The listing builds one solid part. Answer for the finished solid, in the listing's coordinates (mm). Round coordinates to 2 decimals unless told otherwise and drop trailing zeros. Order: outer loops, then holes, each group sorted by start corner. A loop starts at its lowest first (then second) coordinate and runs counter-clockwise, first axis right, second up. Notation, with made-up numbers: (88, -25) -> (135, -25) arc R30 ccw to (135, 13) -> close; hole circle Ø1 at (10, 40). An arc over 180 degrees is marked (long way). Return JSON: item names as keys, results as strings. Group by question number.
(1) The part is cut by section C-C (y = -12). Determine the outline of the cut face in (x, z), plus the area to 3 significant figures.
(2) The part is cut by section A-A (y = 71). Determine the outline of the cut face in (x, z), plus the area to 3 significant figures.
(3) Determine the mould class of faces 1 (the face through (0, 68, 35)), 2 (the face through (3.13, -0.42, -20.64)), 3 (the face through (3.1, 43.4, 131.7)) for opening direction Y: +Y half, -Y half, draft (parallel to the pull), parting line (faces both ways), or undercut.
(4) Consider line 1 (Z direction, x = 1.75, y = 31.75); line 2 (Y direction, x = 2.5, z = -20); line 3 (Z direction, x = 4, y = -31.75). Determine where each line is inside the solid, lowest interval first. Write a range as [from, to].
(5) The part is cut by section B-B (z = 101.5). Determine the outline of the cut face in (x, y), plus the area to 3 significant figures.
(6) Each of these flat-tipped pins is pushed along its axis until it touches: pin 1 (1.5 mm diameter, centred on x = 2.5, y = 41, fed in from -Z); pin 2 (1 mm diameter, centred on x = 4.5, z = 69, fed in from +Y); pin 3 (4 mm diameter, centred on y = 31.75, z = -20.64, fed in from +X); pin 4 (3 mm diameter, centred on x = 2, z = 22, fed in from -Y). Where does it stop, or does it pass through?
Autodesk Inventor part; units mm, degrees
ref_plane "YZ Plane" through (0, 0, 0) normal (1, 0, 0) x (0, 1, 0)
ref_plane "XZ Plane" through (0, 0, 0) normal (0, 1, 0) x (-1, 0, 0)
ref_plane "XY Plane" through (0, 0, 0) normal (0, 0, 1) x (1, 0, 0)
sketch "Sketch1" plane through (0, 0, 0) normal (1, 0, 0) x (0, 1, 0)
  line L0 (31.75, 0) -> (-31.75, 0) construction
  line L1 (-31.75, 0) -> (-31.75, -20.6375) construction
  line L2 (31.75, -20.6375) -> (31.75, 20.6375) construction
  circle A0 centre (31.75, -20.6375) radius 3.175
  circle A1 centre (31.75, 20.6375) radius 3.175
  circle A2 centre (-31.75, -20.6375) radius 3.175
  arc A3 (32.3103, 26.9627) -> (31.75, 121.7883) centre (36.5125, 74.402) ccw
  arc A4 (32.3103, 26.9627) -> (26.7051, 24.4939) centre (31.75, 20.6375) ccw
  arc A5 (-33.2262, -14.4615) -> (-29.3077, -26.499) centre (-31.75, -20.6375) ccw
  arc A6 (-33.2262, -14.4615) -> (26.7051, 24.4939) centre (-58.0173, 89.2573) ccw
  arc A7 (29.3077, -26.499) -> (37.057, -24.1244) centre (31.75, -20.6375) ccw
  arc A8 (29.3077, -26.499) -> (-29.3077, -26.499) centre (0, -96.8375) ccw
  line L3 (51.3987, 74.402) -> (36.5125, 74.402) construction
  arc A9 (52.0189, 132.2442) -> (31.75, 121.7883) centre (48.8804, 113.4545) ccw
  arc A10 (67.5698, 1.3552) -> (52.0189, 132.2442) centre (40.7089, 64.5321) ccw
  line L4 (48.8804, 113.4545) -> (50.8914, 119.8045) construction
  line L5 (67.5698, 1.3552) -> (55.1469, 30.5739) construction
  line L6 (-29.3077, -26.499) -> (-33.2262, -14.4615) construction
  line L7 (31.75, -20.6375) -> (-31.75, -20.6375) construction
  line L8 (25.9987, 99.802) -> (76.7987, 99.802)
  line L9 (76.7987, 99.802) -> (76.7987, 49.002)
  line L10 (76.7987, 49.002) -> (25.9987, 49.002)
  line L11 (25.9987, 49.002) -> (25.9987, 99.802)
  line L12 (25.9987, 99.802) -> (76.7987, 49.002) construction
  line L13 (76.7987, 99.802) -> (25.9987, 49.002) construction
  line L14 (48.8444, 120.4027) -> (52.0189, 132.2442) construction
  arc A11 (67.5698, 1.3552) -> (37.057, -24.1244) centre (94.4307, -61.8218) ccw
  point P0 (0, 0)
  point P1 (0, 0)
  point P2 (51.3987, 74.402)
  point P3 (51.3987, 74.402)
  dimension "d0" = 63.5
  dimension "d1" = 41.275
  dimension "d2" = 6.35
  dimension "d4" = 6.35
  dimension "d6" = 95.25
  dimension "d8" = 4.7625
  dimension "d9" = 19.05
  dimension "d10" = 6.35
  dimension "d12" = 31.75
  dimension "d21" = 50.8
  dimension "d24" = 0.508
extrude "Extrusion1" add sketch "Sketch1" along normal blind 6.35 contours A3 A9 A10 A11 A7 A8 A5 A6 A4
fillet "Fillet2" radius 3.175 1 edges at (3.175, 31.75, 121.7883)
properties part number "climb hook" material "Aluminum 6061"
Answer below:
{
 "1": {"outline": "(0, -21.59) -> (6.35, -21.59) -> (6.35, -6.94) -> (0, -6.94) -> close", "area": "93.0 mm²"},
 "2": {"outline": "(0, 2.93) -> (6.35, 2.93) -> (6.35, 41.56) -> (0, 41.56) -> close; (0, 107.25) -> (6.35, 107.25) -> (6.35, 126.14) -> (0, 126.14) -> close", "area": "365 mm²"},
 "3": {"face 1": "draft", "face 2": "undercut", "face 3": "parting line"},
 "4": {"line 1": "z = [-26.99, -23.81], [-17.46, 17.46], [23.81, 26.99]", "line 2": "y = [-38.07, -34.86], [-28.64, 28.64], [34.86, 39.99]", "line 3": "z = [-26.99, -23.81], [-17.46, -14.1]"},
 "5": {"outline": "(0, 75.68) -> (6.35, 75.68) -> (6.35, 98.56) -> (0, 98.56) -> close", "area": "145 mm²"},
 "6": {"pin 1": "stops at z = -19.66", "pin 2": "stops at y = 109.24", "pin 3": "passes through", "pin 4": "stops at y = 23.5"}
}
